For this review, use the dimensioned drawing (mm, ordinates from the lowest corner) and the shaded views. A direction names the side the tool comes from. Give positions to 0.01 mm unless a question says otherwise; leave off trailing zeros. Write each loop counter-clockwise with the first axis right and the second up, starting at its lowest first coordinate (ties: lowest second). Pieces come first, ordered by that corner, then holes. Notation, with made-up numbers: M -20,-36 L -14,-36 A31 cw -14,-9 Z; hole C -21.75,-28 d7. An arc over 180 degrees is marked long. One line per item, written item: value. Start each with the question number.
Item 1: Consider section C-C, the plane x = 9. Write out the cut boundary in (y, z).
Item 2: Tool access review of the marked faces 1 and 2: name each direction out of +Z, -Z, +X, -X, +Y, -Y from which nothing blocks a thin tool from reaching the whole face with its end or side.
Item 3: Consider section D-D, the plane x = 1.75. Write out the cut boundary in (y, z).
Item 4: To check wall thickness, follow probe 1 along X at (y, z) = (2.25, 2.4); probe 2 along X at (y, z) = (2.15, 4.05); probe 3 along Z at (x, y) = (4, 2.3). State the ranges of each line that lie inside material, in increasing order.
Item 5: Consider section A-A, the plane z = 2.35. Write out the cut boundary in (x, y).
Item 6: Clearance check with flat-ended pins moving along their axes: pin 1 Ø2 at (x, z) = (3, 2) entering from +Y; pin 2 Ø1 at (x, y) = (2.5, 1) entering from +Z; pin 3 Ø0.5 at (x, z) = (9.5, 3.5) entering from +Y. State where each tip first meets the part, or that it passes through.
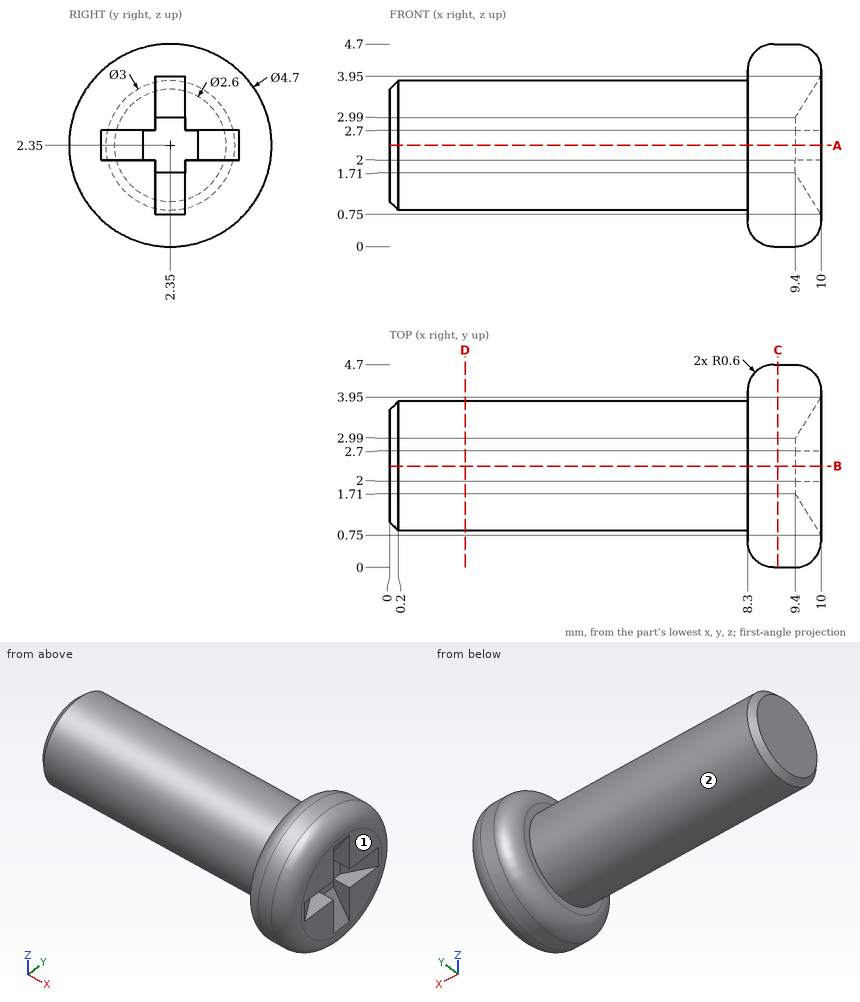
Model answer:
1. outline: C 2.35,2.35 d4.7
2. face 1: +Z, -Z, +X, +Y, -Y
2. face 2: -X
3. outline: C 2.35,2.35 d3
4. probe 1: x = 0 to 9.4
4. probe 2: x = 8.3 to 10
4. probe 3: z = 0.85 to 3.85
5. outline: M 0,1.05 L 0.2,0.85 L 8.3,0.85 L 8.3,0.6 A0.6 ccw 8.9,0 L 9.4,0 A0.6 ccw 10,0.6 L 10,0.75 L 9.4,1.71 L 9.4,2.99 L 10,3.95 L 10,4.1 A0.6 ccw 9.4,4.7 L 8.9,4.7 A0.6 ccw 8.3,4.1 L 8.3,3.85 L 0.2,3.85 L 0,3.65 Z
6. pin 1: stops at y = 3.85
6. pin 2: stops at z = 3.59
6. pin 3: stops at y = 4.52
